Model file for the job. Use its own axes, mm. A direction names the side the tool comes from. Give positions to 0.01 mm unless a question says otherwise; leave off trailing zeros. Loops run counter-clockwise (first coordinate to the right, second up) from the corner with the lowest first, then second, coordinate; pieces in that order, holes last. Notation, with made-up numbers: (4, 54.5) - (19, 54.5) arc R28 cw to (19, 88.5) - close; hole circle Ø2 at (25.5, -3.5). An arc over 180 degrees is marked (long way). Use a Markdown table: item, result.
from build123d import *

# Parameters (mm, degrees)
SKETCH1_R                   = 20
BOSS_EXTRUDE1_DEPTH         = 10
FILLET1_R                   = 6
TAP_DRILL_FOR_M5_TAP1_D     = 4.2
CUT_EXTRUDE2_START          = 5
SKETCH4_OUTSIDE_W           = 97.034
SKETCH4_OUTSIDE_H           = 77.434
SKETCH4_OUTSIDE_W_2         = 56.4
SKETCH4_OUTSIDE_H_2         = 56.4
CUT_EXTRUDE2_DEPTH          = 44.365690319
FILLET2_R                   = 6
FILLET3_R                   = 6
TAP_DRILL_FOR_M5_TAP2_D     = 4.2
TAP_DRILL_FOR_M5_TAP2_DEPTH = 20
TAP_DRILL_FOR_M5_TAP2_TIP   = 1.2618073
BOSS_EXTRUDE2_START         = -6
BOSS_EXTRUDE2_DEPTH         = 3.5
SKETCH10_W                  = 36
SKETCH10_H                  = 49.806381251
CUT_EXTRUDE3_DEPTH          = 2.5
FILLET4_R                   = 4
CHAMFER1_SIZE               = 0.5


with BuildPart() as part:
    # Sketch1 → Boss-Extrude1 (new body)
    with BuildSketch(Plane.XY):
        Polygon((-28.2, -20), (-38, -20), (-38, 20), (-28.2, 20), (-28.2, 28.2), (28.2, 28.2), (28.2, 20), (38, 20), (38, -20), (28.2, -20), (28.2, -28.2), (-28.2, -28.2), align=None)
        Circle(SKETCH1_R, mode=Mode.SUBTRACT)
        with BuildLine():
            Line((-35.559242748, 6), (-35.559242748, 14))
            ThreePointArc((-35.559242748, 14), (-33, 16.559242748), (-30.440757252, 14))
            Line((-30.440757252, 14), (-30.440757252, 6))
            ThreePointArc((-30.440757252, 6), (-33, 3.440757252), (-35.559242748, 6))
        make_face(mode=Mode.SUBTRACT)
        with BuildLine():
            Line((-30.440757252, -6), (-30.440757252, -14))
            ThreePointArc((-30.440757252, -14), (-33, -16.559242748), (-35.559242748, -14))
            Line((-35.559242748, -14), (-35.559242748, -6))
            ThreePointArc((-35.559242748, -6), (-33, -3.440757252), (-30.440757252, -6))
        make_face(mode=Mode.SUBTRACT)
        with BuildLine():
            Line((35.559242748, -6), (35.559242748, -14))
            ThreePointArc((35.559242748, -14), (33, -16.559242748), (30.440757252, -14))
            Line((30.440757252, -14), (30.440757252, -6))
            ThreePointArc((30.440757252, -6), (33, -3.440757252), (35.559242748, -6))
        make_face(mode=Mode.SUBTRACT)
        with BuildLine():
            Line((30.440757252, 6), (30.440757252, 14))
            ThreePointArc((30.440757252, 14), (33, 16.559242748), (35.559242748, 14))
            Line((35.559242748, 14), (35.559242748, 6))
            ThreePointArc((35.559242748, 6), (33, 3.440757252), (30.440757252, 6))
        make_face(mode=Mode.SUBTRACT)
    extrude(amount=BOSS_EXTRUDE1_DEPTH)

    # Fillet1
    fillet1_edges = [part.edges().sort_by_distance(p)[0] for p in [
        (-28.2, 28.2, 5),
        (28.2, 28.2, 5),
        (28.2, -28.2, 5),
        (-28.2, -28.2, 5),
    ]]
    fillet(fillet1_edges, radius=FILLET1_R)

    # Tap Drill for M5 Tap1 (through all)
    with Locations(Plane.XY.offset(10)):
        with Locations((0, 0), (23.57, -23.57), (-23.57, 23.57), (-23.57, -23.57), (23.57, 23.57)):
            Hole(TAP_DRILL_FOR_M5_TAP1_D / 2)

    # Sketch4 outside → Cut-Extrude2 (cut, through all)
    with BuildSketch(Plane(origin=(0, 0, 10), x_dir=(-1, 0, 0), z_dir=(0, 0, -1)).offset(CUT_EXTRUDE2_START)):
        Rectangle(SKETCH4_OUTSIDE_W, SKETCH4_OUTSIDE_H)
        Rectangle(SKETCH4_OUTSIDE_W_2, SKETCH4_OUTSIDE_H_2, mode=Mode.SUBTRACT)
    extrude(amount=CUT_EXTRUDE2_DEPTH, mode=Mode.SUBTRACT)

    # Fillet2
    fillet2_edges = [part.edges().sort_by_distance(p)[0] for p in [
        (38, 20, 7.5),
        (38, -20, 7.5),
        (-38, -20, 7.5),
        (-38, 20, 7.5),
    ]]
    fillet(fillet2_edges, radius=FILLET2_R)

    # Fillet3
    # the kernel refuses this fillet: 6 mm, written as the material it adds along each edge
    with BuildSketch(Plane(origin=(-28.2, -20, 5), x_dir=(0.07169544842088547, -0.9974265700670543, 0), z_dir=(0, 0, 1)), Plane(origin=(28.2, 20, 5), x_dir=(-0.0716954484208838, 0.9974265700670545, 0), z_dir=(0, 0, 1))) as fillet3_piece_1:
        with BuildLine():
            CenterArc((5.486719207, -5.826829434), FILLET3_R, 103.799048999, 64.338369747)
            Line((-0.385141459, -4.593438855), (-0.972327525, -4.470099797))
            ThreePointArc((-0.972327525, -4.470099797), (-0.870898646, -3.747203697), (-0.598455942, 0.043017269))
            Line((-0.598455942, 0.043017269), (0.043017269, 0.598455942))
            ThreePointArc((0.043017269, 0.598455942), (2.237355723, 0.440725956), (3.912504773, 0.582682943))
            Line((3.912504773, 0.582682943), (4.055615176, 0))
        make_face()
    extrude(amount=5)
    with BuildSketch(Plane(origin=(-28.2, 20, 5), x_dir=(-0.9999292752437037, -0.011893044631264506, 0), z_dir=(0, 0, 1)), Plane(origin=(28.2, -20, 5), x_dir=(0.9999292752437039, 0.011893044631263755, 0), z_dir=(0, 0, 1))) as fillet3_piece_2:
        with BuildLine():
            CenterArc((5.348024209, -5.954382082), FILLET3_R, 97.069769939, 64.338369747)
            Line((-0.338858071, -4.04143411), (-0.907546298, -3.850139313))
            ThreePointArc((-0.907546298, -3.850139313), (-0.626122263, -2.192708579), (-0.599957565, 0.007135827))
            Line((-0.599957565, 0.007135827), (0.007135827, 0.599957565))
            ThreePointArc((0.007135827, 0.599957565), (3.806867073, 0.554763996), (4.535710126, 0.595438208))
            Line((4.535710126, 0.595438208), (4.609556861, 0))
        make_face()
    extrude(amount=5)

    # Tap Drill for M5 Tap2
    with Locations(Plane(origin=(0, -28.2, 0), x_dir=(-1, 0, 0), z_dir=(0, -1, 0))):
        with Locations((0, -3.5)):
            Hole(TAP_DRILL_FOR_M5_TAP2_D / 2, depth=TAP_DRILL_FOR_M5_TAP2_DEPTH)
            with Locations((0, 0, -(TAP_DRILL_FOR_M5_TAP2_DEPTH + TAP_DRILL_FOR_M5_TAP2_TIP / 2))):  # 118° drill point
                Cone(0, TAP_DRILL_FOR_M5_TAP2_D / 2, TAP_DRILL_FOR_M5_TAP2_TIP, mode=Mode.SUBTRACT)

    # Sketch9 → Boss-Extrude2 (add)
    with BuildSketch(Plane(origin=(0, 0, 0), x_dir=(-1, 0, 0), z_dir=(0, 0, -1)).offset(BOSS_EXTRUDE2_START)):
        with BuildLine():
            Line((-28.2, 22.2), (-28.2, 34))
            ThreePointArc((-28.2, 34), (-26.442640687, 38.242640687), (-22.2, 40))
            Line((-22.2, 40), (22.2, 40))
            ThreePointArc((22.2, 40), (26.442640687, 38.242640687), (28.2, 34))
            Line((28.2, 34), (28.2, 22.2))
            ThreePointArc((28.2, 22.2), (26.442640687, 26.442640687), (22.2, 28.2))
            Line((22.2, 28.2), (-22.2, 28.2))
            ThreePointArc((-22.2, 28.2), (-26.442640687, 26.442640687), (-28.2, 22.2))
        make_face()
    extrude(amount=BOSS_EXTRUDE2_DEPTH)

    # Sketch10 → Cut-Extrude3 (cut)
    with BuildSketch(Plane(origin=(0, 0, 0), x_dir=(-1, 0, 0), z_dir=(0, 0, -1))):
        with Locations((0, 24.903190626)):
            Rectangle(SKETCH10_W, SKETCH10_H)
    extrude(amount=-CUT_EXTRUDE3_DEPTH, mode=Mode.SUBTRACT)

    # Fillet4
    fillet4_edges = [part.edges().sort_by_distance(p)[0] for p in [
        (-18, 28.2, 1.25),
        (-18, 8.717797887, 1.25),
        (18, 28.2, 1.25),
        (18, 8.717797887, 1.25),
    ]]
    fillet(fillet4_edges, radius=FILLET4_R)

    # Chamfer1
    chamfer1_edges = [part.edges().sort_by_distance(p)[0] for p in [
        (0, -28.2, 10),
        (25.730504921, -27.051343629, 10),
        (-25.730504921, 27.051343629, 10),
        (28.2, 0, 0),
        (25.67, 23.57, 10),
        (25.67, 23.57, 0),
        (-21.47, -23.57, 10),
        (-21.47, -23.57, 0),
        (-21.47, 23.57, 10),
        (-21.47, 23.57, 0),
        (-28.2, 0, 0),
        (25.67, -23.57, 10),
        (25.67, -23.57, 0),
        (38, 0, 10),
        (-38, 0, 10),
        (-36.519700494, -17.946176307, 10),
        (36.519700494, 17.946176307, 10),
        (-25.730504921, -27.051343629, 10),
        (-36.519700494, 17.946176307, 10),
        (25.730504921, 27.051343629, 10),
        (36.519700494, -17.946176307, 10),
        (-29.768125907, -21.28873584, 10),
        (-29.768125907, 21.28873584, 10),
        (29.768125907, 21.28873584, 10),
        (29.768125907, -21.28873584, 10),
        (-33, 3.440757252, 10),
        (-30.440757252, 10, 10),
        (-33, 16.559242748, 10),
        (-35.559242748, 10, 10),
        (-22.1, 28.2, 0),
        (-18, 16.895831523, 0),
        (-4.082482905, -19.578900207, 0),
        (18, 16.895831523, 0),
        (-18.084219959, 8.775166466, 0),
        (18.084219959, 8.775166466, 0),
        (19.171572875, 27.028427125, 0),
        (-19.171572875, 27.028427125, 0),
        (-33, -3.440757252, 10),
        (-35.559242748, -10, 10),
        (-33, -16.559242748, 10),
        (-30.440757252, -10, 10),
        (33, -3.440757252, 10),
        (30.440757252, -10, 10),
        (33, -16.559242748, 10),
        (35.559242748, -10, 10),
        (33, 3.440757252, 10),
        (35.559242748, 10, 10),
        (33, 16.559242748, 10),
        (30.440757252, 10, 10),
        (-20, 0, 10),
        (22.1, 28.2, 0),
        (0, 28.2, 10),
        (0, -28.2, 0),
        (26.442640687, -26.442640687, 0),
        (-26.442640687, -26.442640687, 0),
        (-26.442640687, 26.442640687, 0),
        (26.442640687, 26.442640687, 0),
    ]]
    chamfer(chamfer1_edges, length=CHAMFER1_SIZE)


solid = part.part
(1) Pin check, flat tips, straight feed: P1, Ø1, axis at y = 15, z = 1, coming from the -X side; P2, Ø1.5, axis at y = -15, z = 3.5, coming from the +X side; P3, Ø5, axis at x = 23.57, y = -23.57, coming from the -Z side; P4, Ø4.5, axis at y = 2, z = 3.5, coming from the -X side. Stop position of each tip, or through.
Computed:
| item | result |
|---|---|
| P1 | x = -28.2 |
| P2 | x = 28.2 |
| P3 | z = 0.1 |
| P4 | x = -38 |
(2) Mould opens along Y. For faces 1 (the conical face through (26.228, -26.141, 0.135)), 2 (the flat face through (0, 40, 4)), 3 (the cylindrical face through (33.06, 3.44, 7.22)), 4 (the flat face through (13, -18, 0)) say: pulls with the +Y half, pulls with the -Y half, needs draft (parallel to the pull), parting line crosses it, or undercut.
Computed:
| item | result |
|---|---|
| face 1 | pulls with the -Y half |
| face 2 | pulls with the +Y half |
| face 3 | undercut |
| face 4 | needs draft |
(3) Drill centre lines: probe 1 along Y at (x, z) = (0, 8.75); probe 2 along Y at (x, z) = (25, 1.25); probe 3 along X at (y, z) = (0, 6.75). Where is each one in solid material? Low to high. Write a range as [from, to].
Computed:
| item | result |
|---|---|
| probe 1 | [-28.2, -20], [20, 28.2] |
| probe 2 | [-27.51, -25.11], [-22.03, 22.03], [25.11, 27.51] |
| probe 3 | [-38, -20], [20, 38] |
(4) 3-axis set-ups, long thin cutter, end or side, ignore diameter. For faces 5 (the conical face through (32.94, -3.3, 9.64)), 6 (the cylindrical face through (-32.94, 3.44, 7.22)), 7 (the cylindrical face through (-18.087, 8.764, 1.486)): which of +Z, -Z, +X, -X, +Y, -Y reach the whole face in a straight line?
Computed:
| item | result |
|---|---|
| face 5 | +Z |
| face 6 | +Z, -Z |
| face 7 | -Z |
(5) Slice it at B-B, the plane y = -8.5. Count the separate pieces of the cut face and the enclosed holes in it, plus the area to 3 significant figures.
Computed:
| item | result |
|---|---|
| separate pieces | 4 |
| enclosed holes | 0 |
| area | 247 mm² |
(6) Slice it at A-A, the plane z = 3.5. Write the cut outline in (x, y), plus the area to 3 significant figures.
Computed:
| item | result |
|---|---|
| outline | (-28.2, -22.2) arc R6 ccw to (-22.2, -28.2) - (-2.1, -28.2) - (-2.1, -19.89) arc R20 cw (long way) to (2.1, -19.89) - (2.1, -28.2) - (22.2, -28.2) arc R6 ccw to (28.2, -22.2) - (28.2, 34) arc R6 ccw to (22.2, 40) - (-22.2, 40) arc R6 ccw to (-28.2, 34) - close; hole circle Ø4.2 at (-23.57, -23.57); hole circle Ø4.2 at (-23.57, 23.57); hole circle Ø4.2 at (23.57, -23.57); hole circle Ø4.2 at (23.57, 23.57) |
| area | 2,470 mm² |
